Drawing for the job (mm, zero at the part's lowest x, y, z). A direction names the side the tool comes from. Round coordinates to 2 decimals unless told otherwise and drop trailing zeros. Loops run counter-clockwise (first coordinate to the right, second up) from the corner with the lowest first, then second, coordinate; pieces in that order, holes last. Notation, with made-up numbers: M 81,-6 L 115,-6 A21 ccw 115,4 Z; hole C -14,51 d8. An arc over 180 degrees is marked long. Answer in a Markdown table with one row per item.
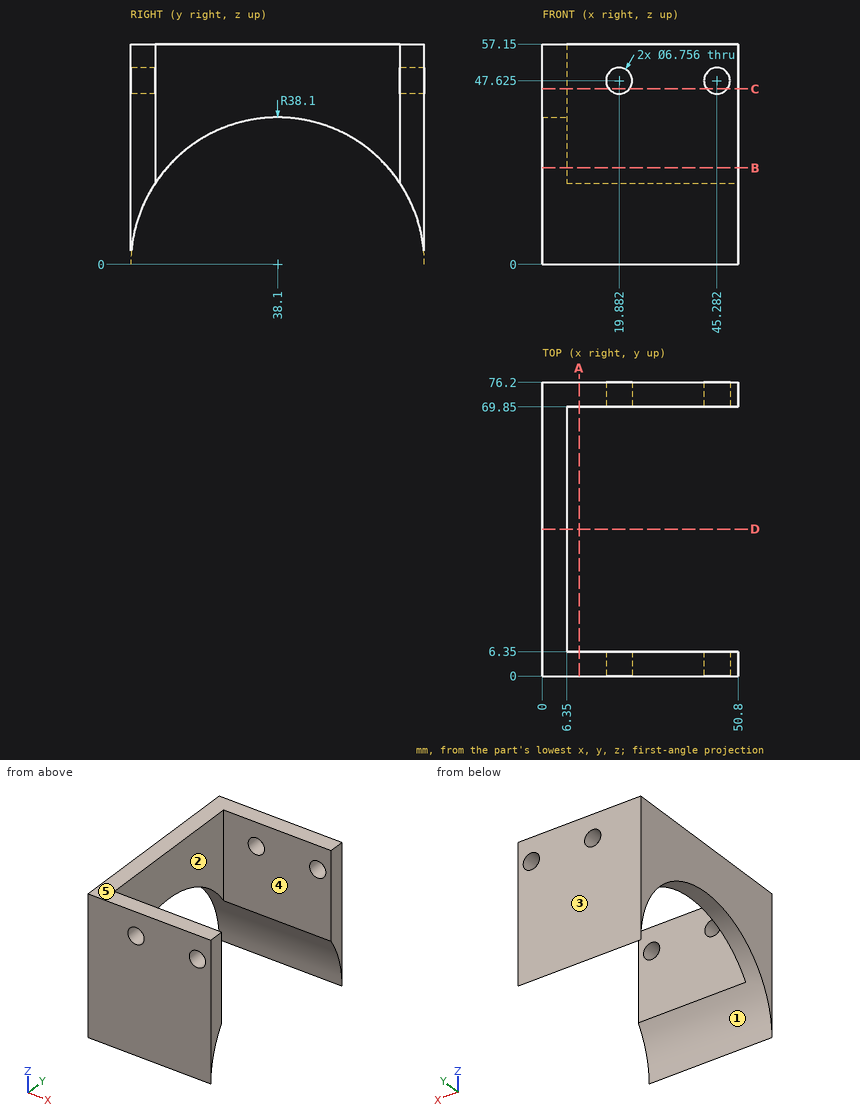
1. Tool access for the marked faces 1 and 2: list every direction of +Z, -Z, +X, -X, +Y, -Y with a clear straight run to the whole face (end or side of a thin tool).
Verdict:
| item | result |
|---|---|
| face 1 | -Z, +X, -X |
| face 2 | +Z, -Z, +X |
2. Mould opens along Y. For the marked faces 3, 4 and 5 say: +Y half, -Y half, draft (parallel to the pull), parting line (faces both ways), or undercut.
Verdict:
| item | result |
|---|---|
| face 3 | +Y half |
| face 4 | undercut |
| face 5 | draft |
3. Saw through at D-D (y = 38.1). Write the cut outline in (x, z), and give its area (3 significant figures).
Verdict:
| item | result |
|---|---|
| outline | M 0,38.1 L 6.35,38.1 L 6.35,57.15 L 0,57.15 Z |
| area | 121 mm² |
4. Saw through at C-C (z = 45.5). State how many separate pieces and enclosed holes the cut face has, and give its area (3 significant figures).
Verdict:
| item | result |
|---|---|
| separate pieces | 5 |
| enclosed holes | 0 |
| area | 915 mm² |
5. Saw through at A-A (x = 9.5). Write the cut outline in (y, z).
Verdict:
| item | result |
|---|---|
| outline | M 0,0 A38.1 cw 6.35,21.06 L 6.35,57.15 L 0,57.15 Z; M 69.85,21.06 A38.1 cw 76.2,0 L 76.2,57.15 L 69.85,57.15 Z |
6. Pin check, flat tips, straight feed: pin 1 (4 mm diameter, centred on x = 45.28, z = 47.62, fed in from +Y); pin 2 (11 mm diameter, centred on y = 24.5, z = 30.5, fed in from +X). Stop position of each tip, or through.
Verdict:
| item | result |
|---|---|
| pin 1 | passes through |
| pin 2 | stops at x = 6.35 |
7. Wall check: probe 1 along Y at (x, z) = (20, 42.5); probe 2 along X at (y, z) = (15.5, 49). Give the ranges that are in metal, low to high.
Verdict:
| item | result |
|---|---|
| probe 1 | y = 0 to 6.35, 69.85 to 76.2 |
| probe 2 | x = 0 to 6.35 |
8. Saw through at B-B (z = 25). Write the cut outline in (x, y), and give its area (3 significant figures).
Verdict:
| item | result |
|---|---|
| outline | M 0,0 L 50.8,0 L 50.8,6.35 L 6.35,6.35 L 6.35,9.35 L 0,9.35 Z; M 0,66.85 L 6.35,66.85 L 6.35,69.85 L 50.8,69.85 L 50.8,76.2 L 0,76.2 Z |
| area | 683 mm² |
